from build123d import *

# Parameters (mm, degrees)
SKETCH_1_R          = 11
EXTRUDE_1_DEPTH     = 18.825
SKETCH_3_R          = 10
CUT_EXTRUDE_1_DEPTH = 17.825
CUT_EXTRUDE_2_DEPTH = 25.420905491
FILLET_1_R          = 0.5
SKETCH_5_W          = 3
SKETCH_5_H          = 0.7
EXTRUDE_2_DEPTH     = 6
FILLET_2_R          = 0.5
SKETCH_7_R          = 3.5
EXTRUDE_3_DEPTH     = 1
SKETCH_8_R          = 1.5
EXTRUDE_4_DEPTH     = 20
CUT_EXTRUDE_START   = -5
CUT_EXTRUDE_3_DEPTH = 5
SKETCH_10_R         = 4
EXTRUDE_5_DEPTH     = 1
FILLET_4_R          = 0.5
CUT_EXTRUDE_START_2 = -0.2
SKETCH_11_R         = 3
SKETCH_11_R_2       = 1.5
CUT_EXTRUDE_4_DEPTH = 0.2
FILLET_5_R          = 0.5


with BuildPart() as part:
    # 草图1 → 凸台-拉伸1 (new, symmetric)
    with BuildSketch(Plane(origin=(0, 0, 0), x_dir=(0, 0, -1), z_dir=(1, 0, 0))):
        with Locations(Location((0, 0, 0), (0, 0, 180))):
            Circle(SKETCH_1_R)
    extrude(amount=EXTRUDE_1_DEPTH, both=True)

    # 草图3 → 切除-拉伸1 (cut, symmetric)
    with BuildSketch(Plane(origin=(0, 0, 0), x_dir=(0, 0, -1), z_dir=(1, 0, 0))):
        Circle(SKETCH_3_R)
    extrude(amount=CUT_EXTRUDE_1_DEPTH, both=True, mode=Mode.SUBTRACT)

    # 草图4 → 切除-拉伸2 (cut, through all)
    with BuildSketch(Plane.XY):
        with BuildLine():
            Line((-10.332925503, 4), (-10.332925503, -4))
            ThreePointArc((-10.332925503, -4), (-11.825, -5.492074497), (-13.317074497, -4))
            Line((-13.317074497, -4), (-13.317074497, 4))
            ThreePointArc((-13.317074497, 4), (-11.825, 5.492074497), (-10.332925503, 4))
        make_face()
    extrude(amount=CUT_EXTRUDE_2_DEPTH, mode=Mode.SUBTRACT)

    # 圆角1
    fillet_1_edges = [part.edges().sort_by_distance(p)[0] for p in [
        (-18.825, 0, -11),
        (18.825, 0, -11),
    ]]
    fillet(fillet_1_edges, radius=FILLET_1_R)

    # 草图5 → 凸台-拉伸2 (add)
    with BuildSketch(Plane.ZY.offset(18.825)):
        with Locations((0, 7)):
            Rectangle(SKETCH_5_W, SKETCH_5_H)
        with Locations((0, -7)):
            Rectangle(SKETCH_5_W, SKETCH_5_H)
    extrude(amount=EXTRUDE_2_DEPTH)

    # 圆角2
    fillet_2_edges = [part.edges().sort_by_distance(p)[0] for p in [
        (-24.825, 7, 1.5),
        (-24.825, 7, -1.5),
        (-24.825, -7, -1.5),
        (-24.825, -7, 1.5),
    ]]
    fillet(fillet_2_edges, radius=FILLET_2_R)

    # 草图7 → 凸台-拉伸3 (add)
    with BuildSketch(Plane(origin=(18.825, 0, 0), x_dir=(0, 0, -1), z_dir=(1, 0, 0))):
        Circle(SKETCH_7_R)
    extrude(amount=EXTRUDE_3_DEPTH)

    # 草图8 → 凸台-拉伸4 (add)
    with BuildSketch(Plane(origin=(19.825, 0, 0), x_dir=(0, 0, -1), z_dir=(1, 0, 0))):
        Circle(SKETCH_8_R)
    extrude(amount=EXTRUDE_4_DEPTH)

    # 草图9 → 切除-拉伸3 (cut)
    with BuildSketch(Plane(origin=(39.825, 0, 0), x_dir=(0, 0, -1), z_dir=(1, 0, 0)).offset(CUT_EXTRUDE_START)):
        with BuildLine():
            Line((-1.019803903, 1.1), (1.019803903, 1.1))
            ThreePointArc((1.019803903, 1.1), (0, 1.5), (-1.019803903, 1.1))
        make_face()
    extrude(amount=CUT_EXTRUDE_3_DEPTH, mode=Mode.SUBTRACT)

    # 草图10 → 凸台-拉伸5 (add)
    with BuildSketch(Plane(origin=(18.825, 0, 0), x_dir=(0, 0, -1), z_dir=(1, 0, 0))):
        Circle(SKETCH_10_R)
    extrude(amount=EXTRUDE_5_DEPTH)

    # 圆角4
    fillet_4_edges = [part.edges().sort_by_distance(p)[0] for p in [
        (19.825, 0, 4),
    ]]
    fillet(fillet_4_edges, radius=FILLET_4_R)

    # 草图11 → 切除-拉伸4 (cut)
    with BuildSketch(Plane(origin=(19.825, 0, 0), x_dir=(0, 0, -1), z_dir=(1, 0, 0)).offset(CUT_EXTRUDE_START_2)):
        Circle(SKETCH_11_R)
        with Locations(Location((0, 0, 0), (0, 0, 132.833428066))):
            Circle(SKETCH_11_R_2, mode=Mode.SUBTRACT)
    extrude(amount=CUT_EXTRUDE_4_DEPTH, mode=Mode.SUBTRACT)

    # 圆角5
    # the kernel refuses this fillet: 0.5 mm, written as the material it takes off along each edge
    with BuildSketch(Plane(origin=(19.825, 0, 0), x_dir=(0, 0, -1), z_dir=(0, -1, 0))) as fillet_5_piece_1:
        with BuildLine():
            CenterArc((3.4, -0.5), FILLET_5_R, 90, 53.130102355)
            Line((3, -0.2), (2.992, -0.194))
            ThreePointArc((2.992, -0.194), (2.99, -0.1), (2.99, 0))
            Line((2.99, 0), (3, 0.01))
            Line((3, 0.01), (3.4, 0.01))
            Line((3.4, 0.01), (3.4, 0))
        make_face()
    revolve(axis=Axis((19.825, 0, 0), (1, 0, 0)), mode=Mode.SUBTRACT)


solid = part.part
Work out the finished part from the listing and answer in its coordinate system (mm). A direction names the side the tool comes from. Coordinates: 2 decimals unless noted, no trailing zeros. Write each loop counter-clockwise with the first axis right and the second up, starting at its lowest first coordinate (ties: lowest second). Pieces come first, ordered by that corner, then holes. Notation, with made-up numbers: M 77.5,-7.75 L 108.5,-7.75 A7 cw 108.5,-0.75 Z; hole C -22.5,35 d8. An arc over 180 degrees is marked long. Use one line per item in the form item = value. Start each with the question number.
1. The part is cut by section A-A (x = 5.5). Give the vertices of the cut face in (y, z).
2. Each of these flat-tipped pins is pushed along its axis until it touches: P1, Ø2.5, axis at x = -21.5, z = 0, coming from the +Y side; P2, Ø0.8, axis at x = -22.5, y = 7, coming from the -Z side; P3, Ø1.5, axis at x = -22.5, z = 0, coming from the -Y side; P4, Ø1.5, axis at y = 8, z = -0.5, coming from the -X side (3 decimals). Where does it stop, or does it pass through?
3. The mould has two halves that part along Z. Classify faces 4 (the face through (-22, -7.35, 0)), 5 (the face through (-17.825, 0, 0)), 6 (the face through (0, 0, -11)): released by +Z, released by -Z, zero draft, split by the parting line, or undercut.
4. Straight lines are drawn through the part: probe 1 along X at (y, z) = (4.5, 5) (3 decimals); probe 2 along X at (y, z) = (3, -2.5) (3 decimals); probe 3 along Y at (x, z) = (-5, 0). For each, find the intervals that lie inside material, in ascending order. Write a range as from..to.
5. A tool of negligible diameter and unlimited length cuts with its end or side. For faces 1 (the face through (18.825, 0, 5)), 2 (the face through (-13.317, -0.1, 10.3)), 3 (the face through (17.825, 0, 0)), from which of +Z, -Z, +X, -X, +Y, -Y can it reach the whole face along a straight path? Write none if from no direction.
Evaluation:
q1.outline = C 0,0 d22; hole C 0,0 d20
q2.P1 = 7.35
q2.P2 = -1.5
q2.P3 = -7.35
q2.P4 = -24.825
q3.face_4 = zero draft
q3.face_5 = undercut
q3.face_6 = split by the parting line
q4.probe_1 = -18.825..-17.825, 17.825..18.825
q4.probe_2 = -18.825..-17.825, 17.825..19.618
q4.probe_3 = -11..-10, 10..11
q5.face_1 = +X
q5.face_2 = +Z
q5.face_3 = none
